Part model, mm, in its own coordinate system. A direction names the side the tool comes from. Round coordinates to 2 decimals unless told otherwise and drop trailing zeros. Loops run counter-clockwise (first coordinate to the right, second up) from the corner with the lowest first, then second, coordinate; pieces in that order, holes last. Notation, with made-up numbers: (-36.5, 85) - (-13.5, 85) arc R9 ccw to (-13.5, 99) - close; hole circle Ø2 at (-6, -21). An arc over 180 degrees is marked (long way). Put each result on its own line as item: value.
Solid Edge part; units mm, degrees
sketch "Sketch1" plane through (0, 0, 0) normal (0, -1, 0) x (1, 0, 0)
  line L0 (-25, 0) -> (25, 0)
  line L1 (25, 0) -> (25, 8.5)
  line L2 (25, 8.5) -> (-25, 8.5)
  line L3 (-25, 8.5) -> (-25, 0)
  dimension "D1" = 25
  dimension "D2" = 25
extrude "Protrusion1" add sketch "Sketch1" against normal blind 36
sketch "Sketch2" plane through (-25, 15, 5) normal (-1, 0, 0) x (0, -1, 0)
  line L0 (-18, 3.5) -> (12, 3.5)
  line L1 (12, 3.5) -> (12, -2)
  line L2 (12, -2) -> (-18, -2)
  line L3 (-18, -2) -> (-18, 3.5)
  dimension "D1" = 18
extrude "Cutout1" cut sketch "Sketch2" against normal through all
sketch "Sketch3" plane through (0, 15, 3) normal (0, 0, 1) x (1, 0, 0)
  circle A0 centre (-18, 3) radius 3
  dimension "D1" = 18
extrude "ExtrudedProtrusion_2" add sketch "Sketch3" along normal blind 4.5
sketch "Sketch4" plane through (0, 15, 0) normal (0, 0, -1) x (1, 0, 0)
  circle A0 centre (-18, -3) radius 2.75
extrude "ExtrudedCutout_2" cut sketch "Sketch4" against normal blind 6.5
sketch "Sketch5" plane through (-15, 15, 7.5) normal (0, 0, 1) x (1, 0, 0)
  circle A0 centre (-3, 3) radius 1.5
extrude "Cutout2" cut sketch "Sketch5" against normal through all
extrude "Cutout3" [suppressed]
extrude "Cutout4" [suppressed]
fillet "Round_1" radius 3 4 edges at (-25, 1.5, 8.5) (-25, 34.5, 8.5) (25, 1.5, 8.5) (25, 34.5, 8.5)
chamfer "Chamfer_1" [suppressed]
hole "Hole_1" at (-14, 0, 5.8) direction (0, 1, 0) diameter 2.5 end up to next countersink diameter 5 countersink angle 90
hole "Hole1" at (3, 0, 5.8) direction (0, 1, 0) diameter 2.5 end up to next countersink diameter 5 countersink angle 90
hole "Hole2" at (20, 0, 5.8) direction (0, 1, 0) diameter 2.5 end up to next countersink diameter 5 countersink angle 90
hole "Hole_4" at (20, 36, 5.8) direction (0, -1, 0) diameter 2.5 end up to next countersink diameter 5 countersink angle 90
hole "Hole3" at (3, 36, 5.8) direction (0, -1, 0) diameter 2.5 end up to next countersink diameter 5 countersink angle 90
hole "Hole4" at (-14, 36, 5.8) direction (0, -1, 0) diameter 2.5 end up to next countersink diameter 5 countersink angle 90
sketch "Sketch6" plane through (0, 18, 3) normal (0, 0, 1) x (1, 0, 0)
  line L0 (-0.5, 12.5) -> (6.5, 12.5)
  line L1 (6.5, 12.5) -> (6.5, 6.5)
  line L2 (6.5, 6.5) -> (-0.5, 6.5)
  line L3 (-0.5, 6.5) -> (-0.5, 12.5)
  line L4 (16.5, 12.5) -> (23.5, 12.5)
  line L5 (23.5, 12.5) -> (23.5, 6.5)
  line L6 (23.5, 6.5) -> (16.5, 6.5)
  line L7 (16.5, 6.5) -> (16.5, 12.5)
  line L8 (23.5, -12.5) -> (16.5, -12.5)
  line L9 (16.5, -12.5) -> (16.5, -6.5)
  line L10 (16.5, -6.5) -> (23.5, -6.5)
  line L11 (23.5, -6.5) -> (23.5, -12.5)
  line L12 (6.5, -12.5) -> (-0.5, -12.5)
  line L13 (-0.5, -12.5) -> (-0.5, -6.5)
  line L14 (-0.5, -6.5) -> (6.5, -6.5)
  line L15 (6.5, -6.5) -> (6.5, -12.5)
  line L16 (-10.5, -12.5) -> (-17.5, -12.5)
  line L17 (-17.5, -12.5) -> (-17.5, -6.5)
  line L18 (-17.5, -6.5) -> (-10.5, -6.5)
  line L19 (-10.5, -6.5) -> (-10.5, -12.5)
  line L20 (-17.5, 12.5) -> (-10.5, 12.5)
  line L21 (-10.5, 12.5) -> (-10.5, 6.5)
  line L22 (-10.5, 6.5) -> (-17.5, 6.5)
  line L23 (-17.5, 6.5) -> (-17.5, 12.5)
  dimension "D1" = 10.5
  dimension "D2" = 10.5
extrude "Cutout5" cut sketch "Sketch6" against normal through all
properties material "ABS Plastic, medium impact"
1. Band-saw the part on C-C (z = 1.5). Give the number of separate pieces and of enclosed holes in the cut face, plus the area to 3 significant figures.
A:
separate pieces: 1
enclosed holes: 7
area: 1,520 mm²
2. Two-plate mould, pull along Y, no slides. Class faces 6 (the flat face through (0, 18, 3)), 7 (the cylindrical face through (-24.14, 1.52, 7.6)), 8 (the flat face through (0, 3, 6)): pulls with the +Y half, pulls with the -Y half, needs draft (parallel to the pull), parting line crosses it, or undercut.
A:
face 6: undercut
face 7: needs draft
face 8: undercut
3. Band-saw the part on A-A (x = -18). List the corners of the cut face in (y, z).
A:
outline: (0, 0) - (15.25, 0) - (15.25, 6.5) - (16.5, 6.5) - (16.5, 7.5) - (15, 7.5) - (15, 3) - (3, 3) - (3, 8.5) - (0, 8.5) - close; (19.5, 6.5) - (20.75, 6.5) - (20.75, 0) - (36, 0) - (36, 8.5) - (33, 8.5) - (33, 3) - (21, 3) - (21, 7.5) - (19.5, 7.5) - close
4. Probe line 1 along Y through (x, z) = (-14.5, 0.5); line 2 along Y through (x, z) = (-18, 6.8); line 3 along Y through (x, z) = (-18, 5.75). List the from-to ranges inside material, lowest first. Write a range as [from, to].
A:
line 1: y = [0, 5.5], [11.5, 24.5], [30.5, 36]
line 2: y = [0, 3], [15, 16.5], [19.5, 21], [33, 36]
line 3: y = [0, 3], [15, 15.25], [20.75, 21], [33, 36]
5. Pin check, flat tips, straight feed: P1, Ø3, axis at x = 9, z = 7, coming from the -Y side; P2, Ø5, axis at x = -19, y = 18, coming from the +Z side; P3, Ø3, axis at x = 20, z = 5.8, coming from the -Y side; P4, Ø1.5, axis at x = 10.5, y = 15, coming from the +Z side. Stop position of each tip, or through.
A:
P1: stops at y = 0
P2: stops at z = 7.5
P3: stops at y = 1
P4: stops at z = 3
6. Band-saw the part on B-B (y = 27). List the corners of the cut face in (x, z), plus the area to 3 significant figures.
A:
outline: (-25, 0) - (-17.5, 0) - (-17.5, 3) - (-25, 3) - close; (-10.5, 0) - (-0.5, 0) - (-0.5, 3) - (-10.5, 3) - close; (6.5, 0) - (16.5, 0) - (16.5, 3) - (6.5, 3) - close; (23.5, 0) - (25, 0) - (25, 3) - (23.5, 3) - close
area: 87.0 mm²
7. Tool access for faces 1 (the cylindrical face through (-12.76, 33.89, 5.64)), 2 (the cylindrical face through (-20.747, 17.879, 3.204)), 3 (the flat face through (25, 18, 2)), 4 (the flat face through (16.5, 27, 2)), 5 (the cylindrical face through (18.78, 33.89, 5.53)): list every direction of +Z, -Z, +X, -X, +Y, -Y with a clear straight run to the whole face (end or side of a thin tool).
A:
face 1: +Y
face 2: -Z
face 3: +Z, -Z, +X, +Y, -Y
face 4: +Z, -Z
face 5: +Y, -Y
8. Band-saw the part on D-D (x = 3). List the corners of the cut face in (y, z), plus the area to 3 significant figures.
A:
outline: (0, 0) - (5.5, 0) - (5.5, 3) - (3, 3) - (3, 4.55) - (1.25, 4.55) - (0, 3.3) - close; (0, 8.3) - (1.25, 7.05) - (3, 7.05) - (3, 8.5) - (0, 8.5) - close; (11.5, 0) - (24.5, 0) - (24.5, 3) - (11.5, 3) - close; (30.5, 0) - (36, 0) - (36, 3.3) - (34.75, 4.55) - (33, 4.55) - (33, 3) - (30.5, 3) - close; (33, 7.05) - (34.75, 7.05) - (36, 8.3) - (36, 8.5) - (33, 8.5) - close
area: 86.9 mm²
